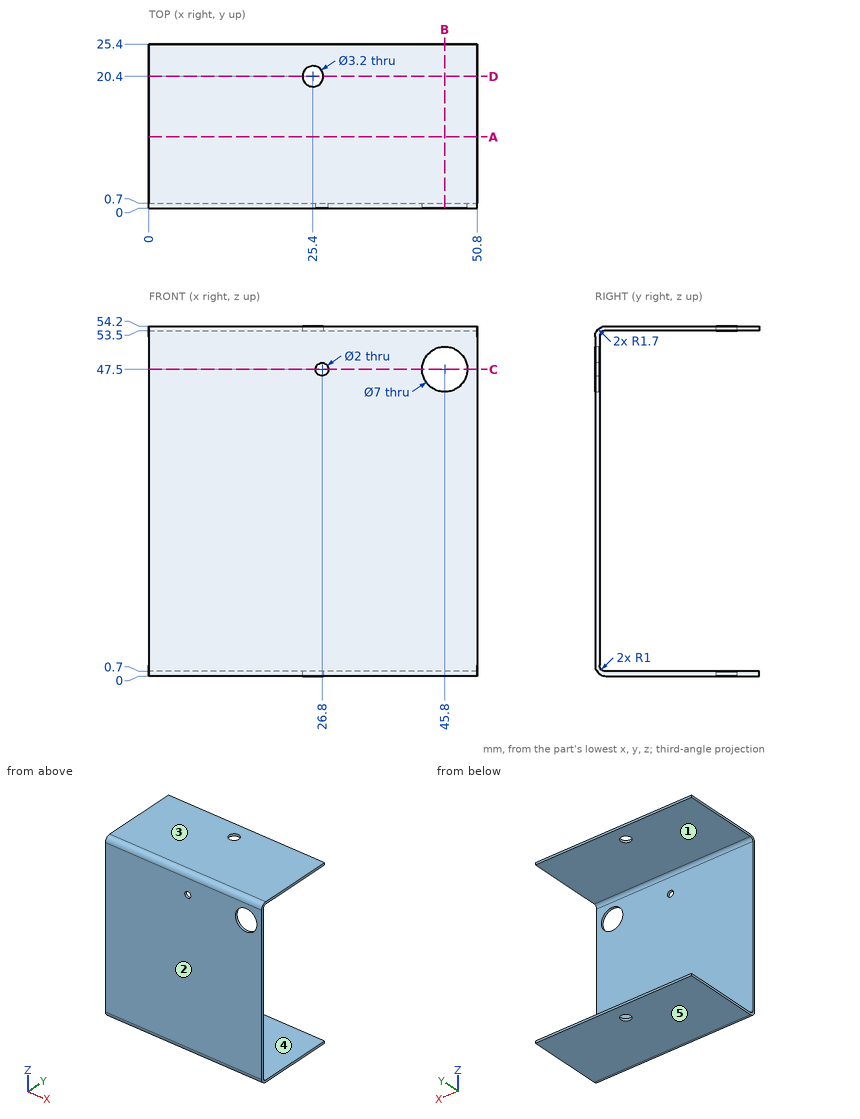
Answer from the drawing. Dimensions are ordinates in mm from the lowest x, y and z of the part. A direction names the side the tool comes from. Round coordinates to 2 decimals unless told otherwise and drop trailing zeros. Write each loop counter-clockwise with the first axis right and the second up, starting at its lowest first coordinate (ties: lowest second). Pieces come first, ordered by that corner, then holes. Notation, with made-up numbers: M 79,5.25 L 92,5.25 A14 ccw 92,10.25 Z; hole C -32,19.5 d9. An arc over 180 degrees is marked long. One line per item, written item: value.
Q1. Flat-ended cylindrical pins translate along their axes: pin 1 Ø8 at (x, z) = (41.5, 48) entering from -Y; pin 2 Ø10 at (y, z) = (9, 26.5) entering from +X; pin 3 Ø4 at (x, z) = (26, 42.5) entering from +Y. Find the tip coordinate at first contact, or state that the pin passes through.
Data:
pin 1: y = 0
pin 2: through
pin 3: y = 0.7
Q2. For a pull along Z with two mould halves and no side action, classify the marked faces 3, 4 and 5 as +Z half, -Z half, draft (parallel to the pull), parting line (faces both ways), or undercut.
Data:
face 3: +Z half
face 4: undercut
face 5: -Z half
Q3. Find section D-D on y = 20.4. Write down the section's boundary in (x, z).
Data:
outline: M 0,0 L 23.8,0 L 23.8,0.7 L 0,0.7 Z; M 0,53.5 L 23.8,53.5 L 23.8,54.2 L 0,54.2 Z; M 27,0 L 50.8,0 L 50.8,0.7 L 27,0.7 Z; M 27,53.5 L 50.8,53.5 L 50.8,54.2 L 27,54.2 Z
Q4. Which of the six approach directions +Z, -Z, +X, -X, +Y, -Y give full straight-line access (tool end or side, diameter ignored) to the marked faces 1 and 2?
Data:
face 1: +X, -X, +Y
face 2: +Z, -Z, +X, -X, -Y
Q5. Straight lines are drawn through the part: line 1 (Z direction, x = 14, y = 7.5); line 2 (X direction, y = 0.25, z = 47.5); line 3 (Y direction, x = 25, z = 32). For each, find the intervals that lie inside material, in ascending order. Write a range as [from, to].
Data:
line 1: [0, 0.7], [53.5, 54.2]
line 2: [0, 25.8], [27.8, 42.3], [49.3, 50.8]
line 3: [0, 0.7]
Q6. Find section A-A on y = 11. Write down the section's boundary in (x, z), plus the area to 3 significant figures.
Data:
outline: M 0,0 L 50.8,0 L 50.8,0.7 L 0,0.7 Z; M 0,53.5 L 50.8,53.5 L 50.8,54.2 L 0,54.2 Z
area: 71.1 mm2
Q7. Find section B-B on x = 45.8. Write down the section's boundary in (y, z).
Data:
outline: M 0,1.7 A1.7 ccw 1.7,0 L 25.4,0 L 25.4,0.7 L 1.7,0.7 A1 cw 0.7,1.7 L 0.7,44 L 0,44 Z; M 0,51 L 0.7,51 L 0.7,52.5 A1 cw 1.7,53.5 L 25.4,53.5 L 25.4,54.2 L 1.7,54.2 A1.7 ccw 0,52.5 Z
Q8. Find section C-C on z = 47.5. Write down the section's boundary in (x, y).
Data:
outline: M 0,0 L 25.8,0 L 25.8,0.7 L 0,0.7 Z; M 27.8,0 L 42.3,0 L 42.3,0.7 L 27.8,0.7 Z; M 49.3,0 L 50.8,0 L 50.8,0.7 L 49.3,0.7 Z
